from build123d import *

# Parameters (mm, degrees)
F1_DEPTH = 63.5
F0_W     = 11.337429
F0_H     = 8.77819
F2_DEPTH = 25.4


with BuildPart() as f1:
    # F0 (on Front) → F1 (new body, symmetric)
    with BuildSketch(Plane.XZ):
        Polygon((32.981567, -26.49961), (32.981567, 26.49961), (13.931567, 26.49961), (-32.981567, 26.49961), (-32.981567, -26.49961), align=None)
    extrude(amount=F1_DEPTH, both=True)

    # F0 (on Front) → F2 (join, symmetric)
    with BuildSketch(Plane.XZ):
        with BuildLine():
            Line((13.931567, 26.49961), (32.981567, 26.49961))
            Line((32.981567, 26.49961), (32.981567, 39.423279))
            ThreePointArc((32.981567, 39.423279), (38.868178, 53.634815), (53.079713, 59.521426))
            Line((53.079713, 59.521426), (68.024464, 59.521426))
            Line((68.024464, 59.521426), (68.024464, 78.571426))
            Line((68.024464, 78.571426), (53.079713, 78.571426))
            ThreePointArc((53.079713, 78.571426), (25.397794, 67.105199), (13.931567, 39.423279))
            Line((13.931567, 39.423279), (13.931567, 26.49961))
        make_face()
        with Locations((73.693178, 82.960521)):
            Rectangle(F0_W, F0_H)
    extrude(amount=F2_DEPTH, both=True)

    # F0 (on Front) → F3 (revolve)
    with BuildSketch(Plane.XZ):
        Polygon((79.361893, 78.571426), (79.361893, 59.521426), (79.361893, 52.306704), (111.312799, 52.306704), (111.312799, 87.349616), (79.361893, 87.349616), align=None)
    revolve(axis=Axis((79.361893, 0, 73.435521), (0, 0, 1)))


solid = f1.part
Geometry check sheet. Reference: the model listing, model coordinates, mm. A direction names the side the tool comes from. Round coordinates to 2 decimals unless told otherwise and drop trailing zeros. Order: outer loops, then holes, each group sorted by start corner. A loop starts at its lowest first (then second) coordinate and runs counter-clockwise, first axis right, second up. Notation, with made-up numbers: M -8.75,0.5 L 34.25,0.5 A32 ccw 34.25,30.5 Z; hole C 60,-31 d10. An arc over 180 degrees is marked long. Answer in a Markdown table with one row per item.
(1) Tool access check on faces 1 (the face through (32, 25.4, 53)), 2 (the face through (55, 23, 59.521)), 3 (the face through (0, -1, 26.5)), 4 (the face through (80, 0, 52.307)). Record the directions out of +Z, -Z, +X, -X, +Y, -Y that give a thin tool (end or side, any length) a straight path to the whole face; none if there is none.
Responses:
| item | result |
|---|---|
| face 1 | +Z, -X, +Y |
| face 2 | -Z, +Y |
| face 3 | +Z, -X |
| face 4 | -Z, +X, +Y, -Y |
(2) Scan lines: probe 1 along Z at (x, y) = (-25.5, -22); probe 2 along X at (y, z) = (20.5, 9); probe 3 along Y at (x, z) = (30.5, 62.5). Record each from-to range of solid material in increasing order. Write a range as from..to.
Responses:
| item | result |
|---|---|
| probe 1 | z = -26.5..26.5 |
| probe 2 | x = -32.98..32.98 |
| probe 3 | y = -25.4..25.4 |
(3) Sectioned sample at B-B, the plane y = -48.5. Record the cut outline in (x, z), and give its area (3 significant figures).
Responses:
| item | result |
|---|---|
| outline | M -32.98,-26.5 L 32.98,-26.5 L 32.98,26.5 L -32.98,26.5 Z |
| area | 3,500 mm² |
(4) Sectioned sample at A-A, the plane z = 54.5. Record the cut outline in (x, y).
Responses:
| item | result |
|---|---|
| outline | M 16.95,-25.4 L 39.79,-25.4 L 39.79,25.4 L 16.95,25.4 Z; C 79.36,0 d63.9 |
(5) Draft check along X on faces 5 (the face through (55, -23, 59.521)), 6 (the face through (55, 23, 78.571)), 7 (the face through (25.704, -0.356, 67.408)). Enter one of: released by +X, released by -X, zero draft, split by the parting line, or undercut.
Responses:
| item | result |
|---|---|
| face 5 | undercut |
| face 6 | zero draft |
| face 7 | released by -X |
(6) Sectioned sample at D-D, the plane z = 7. Record the cut outline in (x, y), and give its area (3 significant figures).
Responses:
| item | result |
|---|---|
| outline | M -32.98,-63.5 L 32.98,-63.5 L 32.98,63.5 L -32.98,63.5 Z |
| area | 8,380 mm² |
(7) Go/stop test with flat-tipped pins: P1, Ø14, axis at x = 37, z = 44, coming from the -Y side; P2, Ø3.5, axis at x = 57, y = -20.5, coming from the -Z side; P3, Ø14, axis at y = -2.5, z = 34, coming from the -X side. Record where each tip stops, or that it passes through.
Responses:
| item | result |
|---|---|
| P1 | stops at y = -25.4 |
| P2 | stops at z = 52.31 |
| P3 | stops at x = 13.93 |
(8) Sectioned sample at C-C, the plane x = 20. Record the cut outline in (y, z).
Responses:
| item | result |
|---|---|
| outline | M -63.5,-26.5 L 63.5,-26.5 L 63.5,26.5 L 25.4,26.5 L 25.4,60.36 L -25.4,60.36 L -25.4,26.5 L -63.5,26.5 Z |
